```python
from build123d import *

# Parameters (mm, degrees)
F1_DEPTH    = 25.4
F3_D        = 25.4
F4_R        = 2.54
F5_T1_DEPTH = 38.1
F5_T4_ANGLE = 90
F5_T6_ANGLE = 90


# Not quite as in the source:
# - a fillet or chamfer that OpenCascade refuses, or shapes differently, is made with other operations: its cross-section is extruded or revolved along the edge and cut away or added


with BuildPart() as f1:
    # F0 (on Top) → F1 (new body)
    with BuildSketch(Plane.XY):
        with BuildLine():
            Line((0, 36.9386635721), (0, 0))
            Line((0, 0), (48.7761497498, 0))
            Line((48.7761497498, 0), (48.7761497498, 36.9386635721))
            ThreePointArc((48.7761497498, 36.9386635721), (24.3880748749, 61.326738447), (0, 36.9386635721))
        make_face()
    extrude(amount=F1_DEPTH)

    # F3 (through all)
    with Locations(Plane.XY.offset(25.4)):
        with Locations((24.3880748749, 36.9386635721)):
            Hole(F3_D / 2)

    # F4
    f4_edges = [f1.edges().sort_by_distance(p)[0] for p in [
        (24.388075, 0, 25.4),
        (48.77615, 18.469332, 25.4),
    ]]
    fillet(f4_edges, radius=F4_R)

    # F5: fillet of radius 5.08 on 2 edges, made by hand

    # F5_s2 → F5_t1 (cut)
    with BuildSketch(Plane.XY.offset(-12.7)):
        with BuildLine():
            ThreePointArc((43.6961497498, 0), (47.2882521982, 1.4878975516), (48.7761497498, 5.08))
            Line((48.7761497498, 5.08), (48.7761497498, 0))
            Line((48.7761497498, 0), (43.6961497498, 0))
        make_face()
        with BuildLine():
            ThreePointArc((0, 5.08), (1.4878975516, 1.4878975516), (5.08, 0))
            Line((5.08, 0), (0, 0))
            Line((0, 0), (0, 5.08))
        make_face()
    extrude(amount=F5_T1_DEPTH, mode=Mode.SUBTRACT)

    # F5_s3 → F5_t4 (revolve, cut)
    with BuildSketch(Plane.XZ.offset(-5.08)):
        with BuildLine():
            ThreePointArc((2.54, 25.4), (0.7439487758, 24.6560512242), (0, 22.86))
            Line((0, 22.86), (0, 25.4))
            Line((0, 25.4), (2.54, 25.4))
        make_face()
    revolve(axis=Axis((5.08, 5.08, 25.4), (0, 0, 1)), revolution_arc=F5_T4_ANGLE, mode=Mode.SUBTRACT)

    # F5_s5 → F5_t6 (revolve, cut)
    with BuildSketch(Plane.YZ.offset(43.6961497498)):
        with BuildLine():
            ThreePointArc((2.54, 25.4), (0.7439487758, 24.6560512242), (0, 22.86))
            Line((0, 22.86), (0, 25.4))
            Line((0, 25.4), (2.54, 25.4))
        make_face()
    revolve(axis=Axis((43.6961497498, 5.08, 25.4), (0, 0, 1)), revolution_arc=F5_T6_ANGLE, mode=Mode.SUBTRACT)


solid = f1.part
```
The model under review builds one solid part; all positions refer to its coordinate system, in mm. Round coordinates to 2 decimals unless told otherwise and drop trailing zeros. Loops run counter-clockwise (first coordinate to the right, second up) from the corner with the lowest first, then second, coordinate; pieces in that order, holes last. Notation, with made-up numbers: (-4, 60) -> (30, 60) arc R33 cw to (30, 95) -> close; hole circle Ø6 at (42, 33). An arc over 180 degrees is marked (long way). Answer as a JSON object with one key per item and string values. Group by question number.
1) We need section A-A on z = 7. Write out the cut boundary in (x, y), then the cut area to 3 significant figures.
2) For pin 1 Ø8 at (x, z) = (17, 21) entering from +Y, flat-tipped, find the tip position at first contact; note if it passes through.
3) For line 1 (Y direction, x = 19.5, z = 15.25); line 2 (X direction, y = 44, z = 18); line 3 (Y direction, x = 34, z = 3.5), list the stretches that pass through material, from the lowest coordinate up. Write a range as [from, to].
4) Mouldability with a two-part tool opening along Y and no side actions: class faces 1 (the face through (24.92, 61.32, 11.27)), 2 (the face through (1.449, 1.528, 11.27)), 3 (the face through (0, 21, 11)), 4 (the face through (12.275, 40.753, 12.522)) as released by +Y, released by -Y, zero draft, split by the parting line, or undercut.
Result set:
{
 "1": {"outline": "(0, 5.08) arc R5.08 ccw to (5.08, 0) -> (43.7, 0) arc R5.08 ccw to (48.78, 5.08) -> (48.78, 36.94) arc R24.39 ccw to (0, 36.94) -> close; hole circle Ø25.4 at (24.39, 36.94)", "area": "2,220 mm²"},
 "2": {"pin 1": "y = 61.09"},
 "3": {"line 1": "[0, 25.22], [48.66, 60.83]", "line 2": "[1.04, 13.83], [34.94, 47.73]", "line 3": "[0, 28.64], [45.24, 59.35]"},
 "4": {"face 1": "released by +Y", "face 2": "released by -Y", "face 3": "zero draft", "face 4": "undercut"}
}
